Build history of the part. All positions in model axes, mm. A direction names the side the tool comes from. Round coordinates to 2 decimals unless told otherwise and drop trailing zeros. Loops run counter-clockwise (first coordinate to the right, second up) from the corner with the lowest first, then second, coordinate; pieces in that order, holes last. Notation, with made-up numbers: (-4, 25.5) - (13, 25.5) arc R12 cw to (13, 33.5) - close; hole circle Ø1 at (-25.5, -19). An arc over 180 degrees is marked (long way). Use a Markdown table: item, result.
from build123d import *

# Parameters (mm, degrees)
CROQUIS1_R              = 7.5
SALIENTE_EXTRUIR1_DEPTH = 12.5
CROQUIS3_R              = 12.5
CROQUIS3_R_2            = 7.5
SALIENTE_EXTRUIR2_DEPTH = 15
CROQUIS4_R              = 17.5
CROQUIS4_R_2            = 7.5
SALIENTE_EXTRUIR3_DEPTH = 2
CROQUIS5_R              = 17.5
CROQUIS5_R_2            = 7.5
SALIENTE_EXTRUIR4_DEPTH = 2


with BuildPart() as part:
    # Croquis1 → Saliente-Extruir1 (new body)
    with BuildSketch(Plane(origin=(0, 0, 0), x_dir=(1, 0, 0), z_dir=(0, 1, 0))):
        with BuildLine():
            Line((-107.423550962, 229), (-89.923550962, 229))
            add(Edge.make_bspline(
                [(-89.923550962, 229), (-92.027233401, 107.676295976), (-12.647886898, 12.09466647)],
                knots=[0, 0, 0, 1, 1, 1], degree=2))
            ThreePointArc((-12.647886898, 12.09466647), (0, 17.5), (12.647886898, 12.09466647))
            add(Edge.make_bspline(
                [(89.923550962, 229), (92.027233401, 107.676295976), (12.647886898, 12.09466647)],
                knots=[0, 0, 0, 1, 1, 1], degree=2))
            Line((89.923550962, 229), (107.423550962, 229))
            add(Edge.make_bspline(
                [(107.423550962, 229), (111.604135582, 83.182199319), (12.139143835, -12.605204756)],
                knots=[0, 0, 0, 1, 1, 1], degree=2))
            ThreePointArc((12.139143835, -12.605204756), (0, -17.5), (-12.139143835, -12.605204756))
            add(Edge.make_bspline(
                [(-107.423550962, 229), (-111.604135582, 83.182199319), (-12.139143835, -12.605204756)],
                knots=[0, 0, 0, 1, 1, 1], degree=2))
        make_face()
        Circle(CROQUIS1_R, mode=Mode.SUBTRACT)
    extrude(amount=SALIENTE_EXTRUIR1_DEPTH)

    # Croquis3 → Saliente-Extruir2 (add, symmetric)
    with BuildSketch(Plane(origin=(98.673550962, 0, 0), x_dir=(0, 0, -1), z_dir=(1, 0, 0))):
        with Locations((236.5, 6.25)):
            Circle(CROQUIS3_R)
        with Locations((236.5, 6.25)):
            Circle(CROQUIS3_R_2, mode=Mode.SUBTRACT)
    saliente_extruir2 = extrude(amount=SALIENTE_EXTRUIR2_DEPTH, both=True)

    # Simetría1: Saliente-Extruir2 across plane
    add(saliente_extruir2.mirror(Plane(origin=(0, 0, 0), x_dir=(0, 0, 1), z_dir=(1, 0, 0))))

    # Croquis4 → Saliente-Extruir3 (add)
    with BuildSketch(Plane(origin=(0, 12.5, 0), x_dir=(1, 0, 0), z_dir=(0, 1, 0))):
        Circle(CROQUIS4_R)
        Circle(CROQUIS4_R_2, mode=Mode.SUBTRACT)
    extrude(amount=SALIENTE_EXTRUIR3_DEPTH)

    # Croquis5 → Saliente-Extruir4 (add)
    with BuildSketch(Plane.XZ):
        Circle(CROQUIS5_R)
        Circle(CROQUIS5_R_2, mode=Mode.SUBTRACT)
    extrude(amount=SALIENTE_EXTRUIR4_DEPTH)


solid = part.part
Q1. Pull direction Z, two halves, no side cores. Call faces 1 (the face through (-98.464, 6.58, -229.007)), 2 (the face through (-76, 12.5, -107)): pulls with the +Z half, pulls with the -Z half, needs draft (parallel to the pull), parting line crosses it, or undercut.
Results found:
| item | result |
|---|---|
| face 1 | undercut |
| face 2 | needs draft |
Q2. Probe line 1 (Y direction, x = 102.25, z = -236.5); line 2 (Z direction, x = 4, y = 4); line 3 (X direction, y = 2.5, z = 0). List the from-to ranges inside material, lowest first.
Results found:
| item | result |
|---|---|
| line 1 | y = -6.25 to -1.25, 13.75 to 18.75 |
| line 2 | z = -17.04 to -6.34, 6.34 to 17.04 |
| line 3 | x = -24.58 to -7.5, 7.5 to 24.58 |
Q3. Cut at A-A, the plane z = -236.5. List the corners of the cut face in (x, y), plus the area to 3 significant figures.
Results found:
| item | result |
|---|---|
| outline | (-113.67, -6.25) - (-83.67, -6.25) - (-83.67, -1.25) - (-113.67, -1.25) - close; (-113.67, 13.75) - (-83.67, 13.75) - (-83.67, 18.75) - (-113.67, 18.75) - close; (83.67, -6.25) - (113.67, -6.25) - (113.67, -1.25) - (83.67, -1.25) - close; (83.67, 13.75) - (113.67, 13.75) - (113.67, 18.75) - (83.67, 18.75) - close |
| area | 600 mm2 |
Q4. Drop flat-ended pins along their axis: pin 1 (2 mm diameter, centred on x = -69, z = -74.5, fed in from +Y); pin 2 (19.5 mm diameter, centred on x = 0, z = 0, fed in from -Y); pin 3 (4 mm diameter, centred on x = 13.5, y = 10, fed in from +Z). Give the stop position or say it passes through.
Results found:
| item | result |
|---|---|
| pin 1 | stops at y = 12.5 |
| pin 2 | stops at y = -2 |
| pin 3 | stops at z = 13.19 |
Q5. Which spindle directions (+Z, -Z, +X, -X, +Y, -Y) get a long thin tool onto all of the face, cutting with end or side? Do faces 3 (the face through (-83.674, -2, -236)), 4 (the face through (0, 14.5, 8)). Say none if no direction does.
Results found:
| item | result |
|---|---|
| face 3 | -Z, +Y, -Y |
| face 4 | +Z, -Z, +X, -X, +Y |
Q6. Cut at B-B, the plane y = 6.25. Count the separate pieces of the cut face and the enclosed holes in it, plus the area to 3 significant figures.
Results found:
| item | result |
|---|---|
| separate pieces | 3 |
| enclosed holes | 1 |
| area | 10,400 mm2 |
